from build123d import *

# Parameters (mm, degrees)
PAD_DEPTH    = 20
SKETCH001_W  = 30
SKETCH001_H  = 18
PAD001_DEPTH = 10
SKETCH002_R  = 1.5
POCKET_DEPTH = 18.001


with BuildPart() as part:
    # Sketch → Pad (new body)
    with BuildSketch(Plane.XY):
        with BuildLine():
            ThreePointArc((-20.838728, 8), (-24.838728, 4), (-20.838728, 0))
            Line((-20.838728, 0), (19.161272, 0))
            ThreePointArc((19.161272, 0), (23.161272, 4), (19.161272, 8))
            Line((-20.838728, 8), (19.161272, 8))
        make_face()
    extrude(amount=PAD_DEPTH)

    # Sketch001 (on Face2 of Pad) → Pad001 (join)
    with BuildSketch(Plane.XZ):
        with Locations((0, 9)):
            Rectangle(SKETCH001_W, SKETCH001_H)
    extrude(amount=PAD001_DEPTH)

    # Sketch002 → Pocket (cut, through all)
    with BuildSketch(Plane(origin=(0, 8, 0), x_dir=(-1, 0, 0), z_dir=(0, 1, 0))):
        with Locations((0, 10)):
            Circle(SKETCH002_R)
    extrude(amount=-POCKET_DEPTH, mode=Mode.SUBTRACT)


solid = part.part
The listing builds one solid part. Answer for the finished solid, in the listing's coordinates (mm). A direction names the side the tool comes from. Round coordinates to 2 decimals unless told otherwise and drop trailing zeros. Write each loop counter-clockwise with the first axis right and the second up, starting at its lowest first coordinate (ties: lowest second). Pieces come first, ordered by that corner, then holes. Notation, with made-up numbers: (46.25, 80) - (65.25, 80) arc R29 cw to (65.25, 106) - close; hole circle Ø3 at (81, -9). An arc over 180 degrees is marked (long way). Use a Markdown table: item, result. Add a question column.
1. The part is cut by section D-D (z = 15.75). Write down the section's boundary in (x, y).
2. The part is cut by section C-C (x = -9.5). Write down the section's boundary in (y, z).
3. Flat-ended cylindrical pins translate along their axes: P1, Ø8, axis at y = -4.5, z = 9, coming from the +X side; P2, Ø2, axis at x = -17, z = 16.5, coming from the -Y side; P3, Ø3, axis at x = 0.5, y = -5, coming from the +Z side. Find the tip coordinate at first contact, or state that the pin passes through.
4. A tool of negligible diameter and unlimited length cuts with its end or side. For faces 1 (the face through (0, -5, 18)), 2 (the face through (-15, -5, 9)), 3 (the face through (-1, 8, 12)), from which of +Z, -Z, +X, -X, +Y, -Y can it reach the whole face along a straight path? Write none if from no direction.
5. The part is cut by section B-B (z = 10). Write down the section's boundary in (x, y), and give its area (3 significant figures).
6. The part is cut by section A-A (x = 0). Write down the section's boundary in (y, z).
7. Consider line 1 (Z direction, x = 0, y = 3.5); line 2 (Z direction, x = 0, y = -3.25); line 3 (Y direction, x = -13, z = 18.5). Determine where each line is inside the solid, lowest interval first.
8. For a pull along X with two mould halves and no side action, classify faces 4 (the face through (-24.838, 4.088, 9.86)), 5 (the face through (15, -5, 9)), 6 (the face through (0.325, -0.874, 8.536)), 7 (the face through (-1, 4, 20)) as +X half, -X half, draft (parallel to the pull), parting line (faces both ways), or undercut.
Reported:
| question | item | result |
|---|---|---|
| 1 | outline | (-20.84, 0) - (-15, 0) - (-15, -10) - (15, -10) - (15, 0) - (19.16, 0) arc R4 ccw to (19.16, 8) - (-20.84, 8) arc R4 ccw to start |
| 2 | outline | (-10, 0) - (8, 0) - (8, 20) - (0, 20) - (0, 18) - (-10, 18) - close |
| 3 | P1 | x = 15 |
| 3 | P2 | y = 0 |
| 3 | P3 | z = 18 |
| 4 | face 1 | +Z, +X, -X, -Y |
| 4 | face 2 | +Z, -Z, -X, -Y |
| 4 | face 3 | +Z, -Z, +X, -X, +Y |
| 5 | outline | (-20.84, 0) - (-15, 0) - (-15, -10) - (-1.5, -10) - (-1.5, 8) - (-20.84, 8) arc R4 ccw to start; (1.5, -10) - (15, -10) - (15, 0) - (19.16, 0) arc R4 ccw to (19.16, 8) - (1.5, 8) - close |
| 5 | area | 616 mm^2 |
| 6 | outline | (-10, 0) - (8, 0) - (8, 8.5) - (-10, 8.5) - close; (-10, 11.5) - (8, 11.5) - (8, 20) - (0, 20) - (0, 18) - (-10, 18) - close |
| 7 | line 1 | 0 to 8.5, 11.5 to 20 |
| 7 | line 2 | 0 to 8.5, 11.5 to 18 |
| 7 | line 3 | 0 to 8 |
| 8 | face 4 | -X half |
| 8 | face 5 | +X half |
| 8 | face 6 | undercut |
| 8 | face 7 | draft |
